Part model, mm, in its own coordinate system. A direction names the side the tool comes from. Round coordinates to 2 decimals unless told otherwise and drop trailing zeros. Loops run counter-clockwise (first coordinate to the right, second up) from the corner with the lowest first, then second, coordinate; pieces in that order, holes last. Notation, with made-up numbers: (-37.75, 12) -> (-24.75, 12) arc R23 cw to (-24.75, 29) -> close; hole circle Ø8 at (58, -22.5). An arc over 180 degrees is marked (long way). Answer as a JSON object with one key per item and string values. Group by question number.
from build123d import *

# Parameters (mm, degrees)
F0_R     = 20
F1_DEPTH = 15
F2_R     = 15
F4_DEPTH = 30
F6_COUNT = 3


with BuildPart() as f1:
    # F0 (on Top) → F1 (new body)
    with BuildSketch(Plane.XY):
        with BuildLine():
            Line((-55, -49.0747728811), (-15, -25.9807621135))
            ThreePointArc((-15, -25.9807621135), (0, -30), (15, -25.9807621135))
            Line((15, -25.9807621135), (55, -49.0747728811))
            Line((55, -49.0747728811), (70, -23.0940107676))
            Line((70, -23.0940107676), (30, 0))
            ThreePointArc((30, 0), (25.9807621135, 15), (15, 25.9807621135))
            Line((15, 25.9807621135), (15, 72.1687836487))
            Line((15, 72.1687836487), (-15, 72.1687836487))
            Line((-15, 72.1687836487), (-15, 25.9807621135))
            ThreePointArc((-15, 25.9807621135), (-25.9807621135, 15), (-30, 0))
            Line((-30, 0), (-70, -23.0940107676))
            Line((-70, -23.0940107676), (-55, -49.0747728811))
        make_face()
        Circle(F0_R, mode=Mode.SUBTRACT)
    extrude(amount=-F1_DEPTH)

    # F2
    f2_edges = [f1.edges().sort_by_distance(p)[0] for p in [
        (-15, 25.980762, -7.5),
        (-30, 0, -7.5),
        (-15, -25.980762, -7.5),
        (15, -25.980762, -7.5),
        (15, 25.980762, -7.5),
        (30, 0, -7.5),
    ]]
    fillet(f2_edges, radius=F2_R)

    # F3 (on face) → F4 (join, through all)
    with BuildSketch(Plane(origin=(7.5, -12.9903810568, 0), x_dir=(0.8660254038, 0.5, 0), z_dir=(0.5, -0.8660254038, 0))):
        Polygon((-72.1687836487, -15), (-72.1687836487, 0), (-95.3969018771, -32.5646207343), (-76.9719982096, -32.5646207343), (-64.4432759996, -15), align=None)
    extrude(amount=-F4_DEPTH)

    # F6: F1 ×3 about axis
    f6_axis = Axis((0, 0, 0.5822554231), (0, 0, -1))


with BuildPart() as f1_1:
    add(f1.part)
    for i in range(1, F6_COUNT):
        add(f1.part.rotate(f6_axis, i * 360 / F6_COUNT))


solid = f1_1.part
Item 1: Which spindle directions (+Z, -Z, +X, -X, +Y, -Y) get a long thin tool onto all of the face, cutting with end or side? Do faces 1 (the face through (-61.21, -35.58, -23.91)), 2 (the face through (-72.31, -41.99, -16.05)). Say none if no direction does.
Item 2: Band-saw the part on D-D, the plane x = 65.5. List the corners of the cut face in (y, z).
Item 3: Drill centre lines: line 1 (Z direction, x = 39, y = -8); line 2 (X direction, y = 63.5, z = -11.5); line 3 (X direction, y = -52, z = -15). Where is each one in solid material? Low to high.
Item 4: Band-saw the part on A-A, the plane x = 0. List the corners of the cut face in (y, z), plus the area to 3 significant figures.
Item 5: Band-saw the part on C-C, the plane y = 0. List the corners of the cut face in (x, z), plus the area to 3 significant figures.
Item 6: Two-plate mould, pull along X, no slides. Class faces 3 (the face through (16.34, 27.34, -7.6)), 4 (the face through (0, -30, -7)), 5 (the face through (-16.34, 27.34, -7.6)), 6 (the face through (61.416, -35.216, -23.905)): pulls with the +X half, pulls with the -X half, needs draft (parallel to the pull), parting line crosses it, or undercut.
Item 7: Drop flat-ended pins along their axis: pin 1 Ø10 at (x, y) = (-34, -39) entering from -Z; pin 2 Ø4.5 at (y, z) = (61.5, -8.5) entering from +X; pin 3 Ø1 at (y, z) = (21, -5) entering from +X. Give the stop position or say it passes through.
Item 8: Band-saw the part on B-B, the plane z = -19. List the corners of the cut face in (x, y), plus the area to 3 significant figures.
Entries:
{
 "1": {"face 1": "-Z, +Y", "face 2": "+Z, -X, -Y"},
 "2": {"outline": "(-55.14, -32.56) -> (-40.49, -32.56) -> (-20.5, -18.55) -> (-20.5, 0) -> (-30.89, 0) -> (-55.14, -17) -> close"},
 "3": {"line 1": "-15 to 0", "line 2": "-15 to 15", "line 3": "-65.67 to -60.07, 60.07 to 65.67"},
 "4": {"outline": "(-30, -15) -> (-20, -15) -> (-20, 0) -> (-30, 0) -> close; (20, -15) -> (64.44, -15) -> (76.97, -32.56) -> (95.4, -32.56) -> (72.17, 0) -> (20, 0) -> close", "area": "1,340 mm²"},
 "5": {"outline": "(-32.21, -15) -> (-20, -15) -> (-20, 0) -> (-32.21, 0) -> close; (20, -15) -> (32.21, -15) -> (32.21, 0) -> (20, 0) -> close", "area": "366 mm²"},
 "6": {"face 3": "pulls with the +X half", "face 4": "undercut", "face 5": "pulls with the -X half", "face 6": "undercut"},
 "7": {"pin 1": "z = -15", "pin 2": "x = 15", "pin 3": "x = 21.9"},
 "8": {"outline": "(-81.74, -29.87) -> (-66.74, -55.85) -> (-50.78, -46.64) -> (-65.78, -20.66) -> close; (-15, 67.3) -> (15, 67.3) -> (15, 85.72) -> (-15, 85.72) -> close; (50.78, -46.64) -> (66.74, -55.85) -> (81.74, -29.87) -> (65.78, -20.66) -> close", "area": "1,660 mm²"}
}
